CAD build for the part. Positions are in the model's coordinates, mm. Round coordinates to 2 decimals unless told otherwise and drop trailing zeros. Order: outer loops, then holes, each group sorted by start corner. A loop starts at its lowest first (then second) coordinate and runs counter-clockwise, first axis right, second up. Notation, with made-up numbers: (-27.5, -10.5) - (1.5, -10.5) arc R14 ccw to (1.5, 14.5) - close; hole circle Ø5 at (31.25, -13). An arc over 180 degrees is marked (long way). Write item = value, one per line.
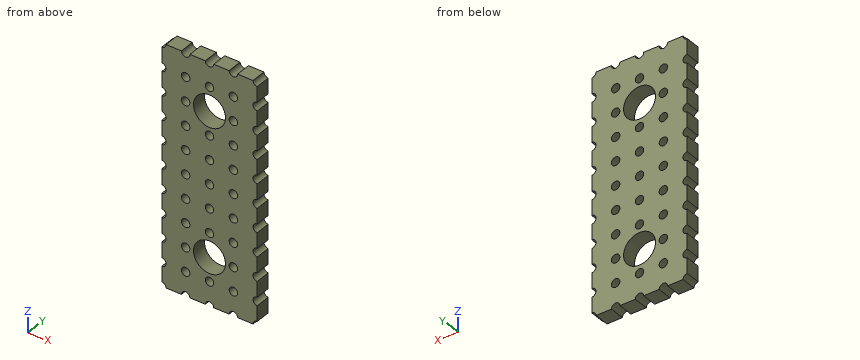
from build123d import *

# Parameters (mm, degrees)
ESQUISSE1_W             = 10.16
ESQUISSE1_H             = 25.4
BOSS_EXTRU_1_DEPTH      = 1.6
ESQUISSE2_R             = 0.45
ENL_V_MAT_EXTRU_1_DEPTH = 23.808828305
D_GAGEMENT_M31_D        = 3.4


with BuildPart() as part:
    # Esquisse1 → Boss.-Extru.1 (new body)
    with BuildSketch(Plane(origin=(0, 0, 0), x_dir=(1, 0, 0), z_dir=(0, 1, 0))):
        with Locations((1.195294118, -9.170147059)):
            Rectangle(ESQUISSE1_W, ESQUISSE1_H)
    extrude(amount=BOSS_EXTRU_1_DEPTH)

    # Esquisse2 → Enlèv. mat.-Extru.1 (cut, through all)
    with BuildSketch(Plane(origin=(0, 1.6, 0), x_dir=(1, 0, 0), z_dir=(0, 1, 0))):
        with Locations((-3.884705882, 3.529852941)):
            Circle(ESQUISSE2_R)
        with Locations((-1.344705882, 3.529852941)):
            Circle(ESQUISSE2_R)
        with Locations((1.195294118, 3.529852941)):
            Circle(ESQUISSE2_R)
        with Locations((3.735294118, 3.529852941)):
            Circle(ESQUISSE2_R)
        with Locations(Location((-1.344705882, 0.989852941, 0), (0, 0, 270))):
            Circle(ESQUISSE2_R)
        with Locations(Location((1.195294118, 0.989852941, 0), (0, 0, 270))):
            Circle(ESQUISSE2_R)
        with Locations(Location((3.735294118, 0.989852941, 0), (0, 0, 270))):
            Circle(ESQUISSE2_R)
        with Locations(Location((-1.344705882, -1.550147059, 0), (0, 0, 270))):
            Circle(ESQUISSE2_R)
        with Locations(Location((1.195294118, -1.550147059, 0), (0, 0, 270))):
            Circle(ESQUISSE2_R)
        with Locations(Location((3.735294118, -1.550147059, 0), (0, 0, 270))):
            Circle(ESQUISSE2_R)
        with Locations(Location((-1.344705882, -4.090147059, 0), (0, 0, 270))):
            Circle(ESQUISSE2_R)
        with Locations(Location((1.195294118, -4.090147059, 0), (0, 0, 270))):
            Circle(ESQUISSE2_R)
        with Locations(Location((3.735294118, -4.090147059, 0), (0, 0, 270))):
            Circle(ESQUISSE2_R)
        with Locations(Location((-1.344705882, -6.630147059, 0), (0, 0, 270))):
            Circle(ESQUISSE2_R)
        with Locations(Location((1.195294118, -6.630147059, 0), (0, 0, 270))):
            Circle(ESQUISSE2_R)
        with Locations(Location((3.735294118, -6.630147059, 0), (0, 0, 270))):
            Circle(ESQUISSE2_R)
        with Locations(Location((-1.344705882, -9.170147059, 0), (0, 0, 270))):
            Circle(ESQUISSE2_R)
        with Locations(Location((1.195294118, -9.170147059, 0), (0, 0, 270))):
            Circle(ESQUISSE2_R)
        with Locations(Location((3.735294118, -9.170147059, 0), (0, 0, 270))):
            Circle(ESQUISSE2_R)
        with Locations(Location((-1.344705882, -11.710147059, 0), (0, 0, 270))):
            Circle(ESQUISSE2_R)
        with Locations(Location((1.195294118, -11.710147059, 0), (0, 0, 270))):
            Circle(ESQUISSE2_R)
        with Locations(Location((3.735294118, -11.710147059, 0), (0, 0, 270))):
            Circle(ESQUISSE2_R)
        with Locations(Location((-1.344705882, -14.250147059, 0), (0, 0, 270))):
            Circle(ESQUISSE2_R)
        with Locations(Location((1.195294118, -14.250147059, 0), (0, 0, 270))):
            Circle(ESQUISSE2_R)
        with Locations(Location((3.735294118, -14.250147059, 0), (0, 0, 270))):
            Circle(ESQUISSE2_R)
        with Locations((-3.884705882, 0.989852941)):
            Circle(ESQUISSE2_R)
        with Locations((-3.884705882, -1.550147059)):
            Circle(ESQUISSE2_R)
        with Locations((-3.884705882, -4.090147059)):
            Circle(ESQUISSE2_R)
        with Locations((-3.884705882, -6.630147059)):
            Circle(ESQUISSE2_R)
        with Locations((-3.884705882, -9.170147059)):
            Circle(ESQUISSE2_R)
        with Locations((-3.884705882, -11.710147059)):
            Circle(ESQUISSE2_R)
        with Locations((-3.884705882, -14.250147059)):
            Circle(ESQUISSE2_R)
        with Locations((6.275294118, 3.529852941)):
            Circle(ESQUISSE2_R)
        with Locations((6.275294118, 0.989852941)):
            Circle(ESQUISSE2_R)
        with Locations((6.275294118, -1.550147059)):
            Circle(ESQUISSE2_R)
        with Locations((6.275294118, -4.090147059)):
            Circle(ESQUISSE2_R)
        with Locations((6.275294118, -6.630147059)):
            Circle(ESQUISSE2_R)
        with Locations((6.275294118, -9.170147059)):
            Circle(ESQUISSE2_R)
        with Locations((6.275294118, -11.710147059)):
            Circle(ESQUISSE2_R)
        with Locations((6.275294118, -14.250147059)):
            Circle(ESQUISSE2_R)
        with Locations((-3.884705882, -16.790147059)):
            Circle(ESQUISSE2_R)
        with Locations(Location((-1.344705882, -16.790147059, 0), (0, 0, 270))):
            Circle(ESQUISSE2_R)
        with Locations(Location((1.195294118, -16.790147059, 0), (0, 0, 270))):
            Circle(ESQUISSE2_R)
        with Locations(Location((3.735294118, -16.790147059, 0), (0, 0, 270))):
            Circle(ESQUISSE2_R)
        with Locations((6.275294118, -16.790147059)):
            Circle(ESQUISSE2_R)
        with Locations((-3.884705882, -19.330147059)):
            Circle(ESQUISSE2_R)
        with Locations(Location((-1.344705882, -19.330147059, 0), (0, 0, 270))):
            Circle(ESQUISSE2_R)
        with Locations(Location((1.195294118, -19.330147059, 0), (0, 0, 270))):
            Circle(ESQUISSE2_R)
        with Locations(Location((3.735294118, -19.330147059, 0), (0, 0, 270))):
            Circle(ESQUISSE2_R)
        with Locations((6.275294118, -19.330147059)):
            Circle(ESQUISSE2_R)
        with Locations((-3.884705882, -21.870147059)):
            Circle(ESQUISSE2_R)
        with Locations((-1.344705882, -21.870147059)):
            Circle(ESQUISSE2_R)
        with Locations((1.195294118, -21.870147059)):
            Circle(ESQUISSE2_R)
        with Locations((3.735294118, -21.870147059)):
            Circle(ESQUISSE2_R)
        with Locations((6.275294118, -21.870147059)):
            Circle(ESQUISSE2_R)
    extrude(amount=-ENL_V_MAT_EXTRU_1_DEPTH, mode=Mode.SUBTRACT)

    # Dégagement M31 (through all)
    with Locations(Plane(origin=(0, 1.6, 0), x_dir=(1, 0, 0), z_dir=(0, 1, 0))):
        with Locations((1.195294118, -16.790147059), (1.195294118, -1.550147059)):
            Hole(D_GAGEMENT_M31_D / 2)


solid = part.part
(1) Probe line 1 along Z through (x, y) = (0, 0.9); line 2 along X through (y, z) = (1.45, 19.5); line 3 along X through (y, z) = (1.45, 16.5). List the from-to ranges inside material, lowest first.
Solved:
line_1 = -3.53 to 0.34, 2.76 to 15.58, 18 to 21.87
line_2 = -3.47 to -1.76, -0.93 to 0.78, 1.61 to 3.32, 4.15 to 5.86
line_3 = -3.54 to -1.69, -1 to -0.48, 2.87 to 3.39, 4.08 to 5.93
(2) Band-saw the part on C-C on z = 2.25. List the corners of the cut face in (x, y).
Solved:
outline = (-3.88, 0) - (-0.35, 0) - (-0.35, 1.6) - (-3.88, 1.6) - close; (2.74, 0) - (6.28, 0) - (6.28, 1.6) - (2.74, 1.6) - close
(3) Band-saw the part on A-A on z = 18. List the corners of the cut face in (x, y), plus the area to 3 significant figures.
Solved:
outline = (-3.88, 0) - (0, 0) - (0, 1.6) - (-3.88, 1.6) - close; (2.39, 0) - (6.28, 0) - (6.28, 1.6) - (2.39, 1.6) - close
area = 12.4 mm²
(4) Band-saw the part on B-B on x = 2. List the corners of the cut face in (y, z), plus the area to 3 significant figures.
Solved:
outline = (0, -3.53) - (1.6, -3.53) - (1.6, 0.05) - (0, 0.05) - close; (0, 3.05) - (1.6, 3.05) - (1.6, 15.29) - (0, 15.29) - close; (0, 18.29) - (1.6, 18.29) - (1.6, 21.87) - (0, 21.87) - close
area = 31.1 mm²
(5) Band-saw the part on D-D on y = 0.85. Count the separate pieces of the cut face and the enclosed holes in it, plus the area to 3 significant figures.
Solved:
separate_pieces = 1
enclosed_holes = 27
area = 216 mm²
